The listing builds one solid part. Answer for the finished solid, in the listing's coordinates (mm). Round coordinates to 2 decimals unless told otherwise and drop trailing zeros. Order: outer loops, then holes, each group sorted by start corner. A loop starts at its lowest first (then second) coordinate and runs counter-clockwise, first axis right, second up. Notation, with made-up numbers: (44.25, 82) -> (48.25, 82) arc R35 cw to (48.25, 117) -> close; hole circle Ø1 at (76.25, 24.5). An arc over 180 degrees is marked (long way). Answer in a Markdown table with one row per item. Add a question column.
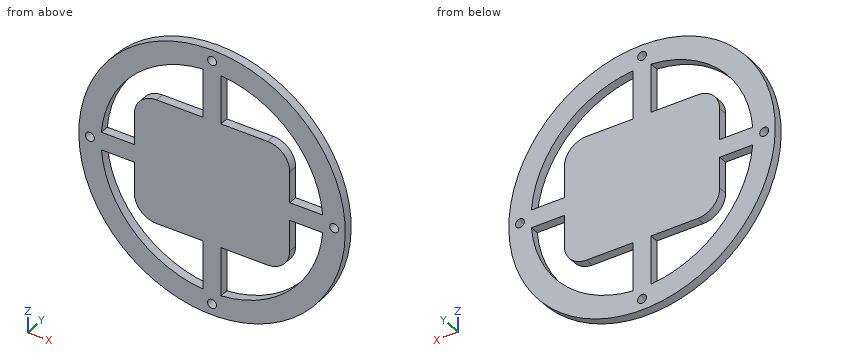
```python
from build123d import *

# Parameters (mm, degrees)
SKETCH1_R           = 30
SKETCH1_R_2         = 25
BOSS_EXTRUDE1_DEPTH = 2
SKETCH2_R           = 1
CUT_EXTRUDE1_DEPTH  = 2
BOSS_EXTRUDE2_DEPTH = 2
FILLET1_R           = 5


with BuildPart() as part:
    # Sketch1 → Boss-Extrude1 (new body)
    with BuildSketch(Plane(origin=(0, 0, 0), x_dir=(1, 0, 0), z_dir=(0, 1, 0))):
        with Locations(Location((0, 0, 0), (0, 0, 270))):
            Circle(SKETCH1_R)
        with Locations(Location((0, 0, 0), (0, 0, 270))):
            Circle(SKETCH1_R_2, mode=Mode.SUBTRACT)
    extrude(amount=BOSS_EXTRUDE1_DEPTH)

    # Sketch2 → Cut-Extrude1 (cut)
    with BuildSketch(Plane(origin=(0, 2, 0), x_dir=(1, 0, 0), z_dir=(0, 1, 0))):
        with Locations(Location((0, 27.5, 0), (0, 0, 270))):
            Circle(SKETCH2_R)
        with Locations(Location((27.5, 0, 0), (0, 0, 270))):
            Circle(SKETCH2_R)
        with Locations(Location((0, -27.5, 0), (0, 0, 270))):
            Circle(SKETCH2_R)
        with Locations(Location((-27.5, 0, 0), (0, 0, 270))):
            Circle(SKETCH2_R)
    extrude(amount=-CUT_EXTRUDE1_DEPTH, mode=Mode.SUBTRACT)

    # Sketch3 → Boss-Extrude2 (add)
    with BuildSketch(Plane(origin=(0, 0, 0), x_dir=(1, 0, 0), z_dir=(0, 1, 0))):
        with BuildLine():
            Line((17.5, 14), (2, 14))
            Line((2, 14), (2, 24.919871589))
            ThreePointArc((2, 24.919871589), (0, 25), (-2, 24.919871589))
            Line((-2, 24.919871589), (-2, 14))
            Line((-2, 14), (-17.5, 14))
            Line((-17.5, 14), (-17.5, 2))
            Line((-17.5, 2), (-24.919871589, 2))
            ThreePointArc((-24.919871589, 2), (-25, 0), (-24.919871589, -2))
            Line((-24.919871589, -2), (-17.5, -2))
            Line((-17.5, -2), (-17.5, -14))
            Line((-17.5, -14), (-2, -14))
            Line((-2, -14), (-2, -24.919871589))
            ThreePointArc((-2, -24.919871589), (0, -25), (2, -24.919871589))
            Line((2, -24.919871589), (2, -14))
            Line((2, -14), (17.5, -14))
            Line((17.5, -14), (17.5, -2))
            Line((17.5, -2), (24.919871589, -2))
            ThreePointArc((24.919871589, -2), (25, 0), (24.919871589, 2))
            Line((24.919871589, 2), (17.5, 2))
            Line((17.5, 2), (17.5, 14))
        make_face()
    extrude(amount=BOSS_EXTRUDE2_DEPTH)

    # Fillet1
    fillet1_edges = [part.edges().sort_by_distance(p)[0] for p in [
        (-17.5, 1, 14),
        (17.5, 1, 14),
        (17.5, 1, -14),
        (-17.5, 1, -14),
    ]]
    fillet(fillet1_edges, radius=FILLET1_R)


solid = part.part
```
1. Each of these flat-tipped pins is pushed along its axis until it touches: pin 1 (1 mm diameter, centred on x = -5, y = 1, fed in from -Z); pin 2 (1 mm diameter, centred on y = 0.5, z = -4.5, fed in from -X); pin 3 (0.6 mm diameter, centred on x = 23, y = 0.5, fed in from +Z); pin 4 (1.6 mm diameter, centred on x = -27.5, z = 0, fed in from +Y). Where does it stop, or does it pass through?
2. Straight lines are drawn through the part: line 1 along X through (y, z) = (1.5, 0); line 2 along Z through (x, y) = (9, 0.4); line 3 along Z through (x, y) = (15, 0.95). For each, find the intervals that lie inside material, in ascending order.
3. The part is cut by section D-D (x = 27.5). Give the vertices of the cut face in (y, z), then the cut area to 3 significant figures.
4. The part is cut by section C-C (y = 1.5). Give the number of separate pieces and of enclosed holes in the cut face, then the cut area to 3 significant figures.
5. The part is cut by section A-A (z = 0). Give the vertices of the cut face in (x, y), then the cut area to 3 significant figures.
6. The part is cut by section B-B (x = 16). Give the vertices of the cut face in (y, z), then the cut area to 3 significant figures.
Report:
| question | item | result |
|---|---|---|
| 1 | pin 1 | stops at z = -29.66 |
| 1 | pin 2 | stops at x = -29.73 |
| 1 | pin 3 | stops at z = 19.61 |
| 1 | pin 4 | passes through |
| 2 | line 1 | x = -30 to -28.5, -26.5 to 26.5, 28.5 to 30 |
| 2 | line 2 | z = -28.62 to -23.32, -14 to 14, 23.32 to 28.62 |
| 2 | line 3 | z = -25.98 to -20, -13.33 to 13.33, 20 to 25.98 |
| 3 | outline | (0, -11.99) -> (2, -11.99) -> (2, -1) -> (0, -1) -> close; (0, 1) -> (2, 1) -> (2, 11.99) -> (0, 11.99) -> close |
| 3 | area | 44.0 mm^2 |
| 4 | separate pieces | 1 |
| 4 | enclosed holes | 8 |
| 4 | area | 1,960 mm^2 |
| 5 | outline | (-30, 0) -> (-28.5, 0) -> (-28.5, 2) -> (-30, 2) -> close; (-26.5, 0) -> (26.5, 0) -> (26.5, 2) -> (-26.5, 2) -> close; (28.5, 0) -> (30, 0) -> (30, 2) -> (28.5, 2) -> close |
| 5 | area | 112 mm^2 |
| 6 | outline | (0, -25.38) -> (2, -25.38) -> (2, -19.21) -> (0, -19.21) -> close; (0, -12.57) -> (2, -12.57) -> (2, 12.57) -> (0, 12.57) -> close; (0, 19.21) -> (2, 19.21) -> (2, 25.38) -> (0, 25.38) -> close |
| 6 | area | 75.0 mm^2 |
